Model file for the job. Use its own axes, mm. A direction names the side the tool comes from. Coordinates: 2 decimals unless noted, no trailing zeros. Order: outer loops, then holes, each group sorted by start corner. A loop starts at its lowest first (then second) coordinate and runs counter-clockwise, first axis right, second up. Notation, with made-up numbers: (51, 49) -> (84, 49) arc R9 ccw to (84, 57) -> close; hole circle Ø1 at (46, 72.5). An arc over 180 degrees is marked (long way). Write item = value, one per line. Start each with the question number.
Q1. Cut at D-D, the plane z = 0.75. Give the number of separate pieces and of enclosed holes in the cut face, plus the area to 3 significant figures.
Q2. Cut at A-A, the plane y = -10. List the corners of the cut face in (x, z), plus the area to 3 significant figures.
Q3. 3-axis set-ups, long thin cutter, end or side, ignore diameter. For faces 5 (the face through (-38, -11, 2)), 6 (the face through (-44, 28, 2)), 7 (the face through (-1, 36, 2)): which of +Z, -Z, +X, -X, +Y, -Y reach the whole face in a straight line?
Q4. Mould opens along X. For faces 1 (the face through (-43, -11, 2)), 2 (the face through (-1, -36, 2)), 3 (the face through (-44.46, -25.76, 3.01)), 4 (the face through (-51, -1, 1)) say: +X half, -X half, draft (parallel to the pull), parting line (faces both ways), or undercut.
Q5. Flat gauge pins, fed straight in: pin 1 (10 mm diameter, centred on x = 11, y = -11.5, fed in from -Z); pin 2 (1.4 mm diameter, centred on y = -1.5, z = 3.5, fed in from -X); pin 3 (3 mm diameter, centred on x = -45.75, y = 26.75, fed in from -Z) (3 decimals); pin 4 (0.6 mm diameter, centred on x = 50.5, y = 0.5, fed in from +Z). Where does each tip first touch, or does it go through?
Q6. Cut at B-B, the plane x = -40.5. List the corners of the cut face in (y, z) (3 decimals).
Q7. Cut at C-C, the plane y = -26.75. List the corners of the cut face in (x, z) (3 decimals), plus the area to 3 significant figures.
Q8. Wall check: line 1 (Y direction, x = -40.5, z = 1.05) (3 decimals); line 2 (Y direction, x = -45.75, z = 2.9) (3 decimals); line 3 (X direction, y = -27, z = 0.4). Give the ranges that are in metal, low to high. Write a range as from..to.
from build123d import *

# Parameters (mm, degrees)
F0_W           = 102
F0_H           = 72
F1_DEPTH       = 2.75
F2_W           = 99.5
F2_H           = 72
F3_DEPTH       = 1.25
F5_D           = 3.25
F5_DEPTH       = 8
F5_CBORE_D     = 6
F5_CBORE_DEPTH = 2
F7_DEPTH       = 4
F9_D           = 2.25
F11_D          = 12


with BuildPart() as f1:
    # F0 (on Top) → F1 (new body)
    with BuildSketch(Plane.XY):
        Rectangle(F0_W, F0_H)
    extrude(amount=F1_DEPTH)

    # F2 (on face) → F3 (join)
    with BuildSketch(Plane.XY.offset(2.75)):
        Rectangle(F2_W, F2_H)
    extrude(amount=F3_DEPTH)

    # F5
    with Locations(Plane(origin=(0, 0, 0), x_dir=(1, 0, 0), z_dir=(0, 0, -1))):
        with Locations((-45.75, 26.75), (45.75, 26.75), (45.75, -26.75), (-45.75, -26.75)):
            CounterBoreHole(F5_D / 2, F5_CBORE_D / 2, F5_CBORE_DEPTH, depth=F5_DEPTH)

    # F6 (on face) → F7 (cut)
    with BuildSketch(Plane(origin=(0, 0, 0), x_dir=(1, 0, 0), z_dir=(0, 0, -1))):
        Polygon((-40.5, 16), (-43, 16), (-43, 6), (-40.5, 6), (-38, 6), (-38, 11), (-38, 16), align=None)
    extrude(amount=-F7_DEPTH, mode=Mode.SUBTRACT)

    # F9 (through all)
    with Locations(Plane(origin=(0, 0, 0), x_dir=(1, 0, 0), z_dir=(0, 0, -1))):
        with Locations((-40.5, 20.5), (-40.5, 1.5)):
            Hole(F9_D / 2)

    # F11 (through all)
    with Locations(Plane(origin=(0, 0, 0), x_dir=(1, 0, 0), z_dir=(0, 0, -1))):
        with Locations((0, -24)):
            Hole(F11_D / 2)


solid = f1.part
Here are the results:
q1.separate_pieces = 1
q1.enclosed_holes = 8
q1.area = 7,060 mm²
q2.outline = (-51, 0) -> (-43, 0) -> (-43, 4) -> (-49.75, 4) -> (-49.75, 2.75) -> (-51, 2.75) -> close; (-38, 0) -> (51, 0) -> (51, 2.75) -> (49.75, 2.75) -> (49.75, 4) -> (-38, 4) -> close
q2.area = 385 mm²
q3.face_5 = +Z, -Z
q3.face_6 = -Z
q3.face_7 = +Z, -Z, +X, -X, +Y
q4.face_1 = undercut
q4.face_2 = draft
q4.face_3 = undercut
q4.face_4 = -X half
q5.pin_1 = 0
q5.pin_2 = -49.75
q5.pin_3 = through
q5.pin_4 = 2.75
q6.outline = (-36, 0) -> (-21.625, 0) -> (-21.625, 4) -> (-36, 4) -> close; (-19.375, 0) -> (-16, 0) -> (-16, 4) -> (-19.375, 4) -> close; (-6, 0) -> (-2.625, 0) -> (-2.625, 4) -> (-6, 4) -> close; (-0.375, 0) -> (36, 0) -> (36, 4) -> (-0.375, 4) -> close
q7.outline = (-51, 0) -> (-48.75, 0) -> (-48.75, 2) -> (-47.375, 2) -> (-47.375, 4) -> (-49.75, 4) -> (-49.75, 2.75) -> (-51, 2.75) -> close; (-44.125, 2) -> (-42.75, 2) -> (-42.75, 0) -> (42.75, 0) -> (42.75, 2) -> (44.125, 2) -> (44.125, 4) -> (-44.125, 4) -> close; (47.375, 2) -> (48.75, 2) -> (48.75, 0) -> (51, 0) -> (51, 2.75) -> (49.75, 2.75) -> (49.75, 4) -> (47.375, 4) -> close
q7.area = 368 mm²
q8.line_1 = -36..-21.625, -19.375..-16, -6..-2.625, -0.375..36
q8.line_2 = -36..-28.375, -25.125..25.125, 28.375..36
q8.line_3 = -51..-48.74, -42.76..42.76, 48.74..51
